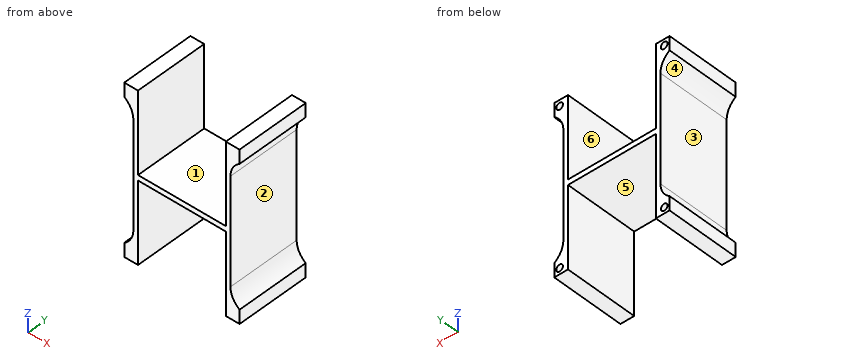
```python
from build123d import *

# Parameters (mm, degrees)
ESQUISSE1_W                  = 43
ESQUISSE1_H                  = 43
BOSS_EXTRU_1_DEPTH           = 40
ESQUISSE2_W                  = 48
ESQUISSE2_H                  = 48
BOSS_EXTRU_2_DEPTH           = 1.5
ENL_V_MAT_EXTRU_3_REACH      = 79.293
ESQUISSE5_W                  = 8
ESQUISSE5_H                  = 5
ENL_V_MAT_EXTRU_4_REACH      = 78.569
ESQUISSE6_W                  = 54.781223227
ESQUISSE6_H                  = 3.078773465
ENL_V_MAT_EXTRU_5_DEPTH      = 9.5
ENL_V_MAT_EXTRU_6_DEPTH      = 73.216687822
ENL_V_MAT_EXTRU_6_DEPTH_BACK = 73.216687822
ESQUISSE9_W                  = 82.255914314
ESQUISSE9_H                  = 90.950558943
ENL_V_MAT_EXTRU_7_DEPTH      = 9.5
ESQUISSE10_W                 = 6
ESQUISSE10_H                 = 36
BOSS_EXTRU_3_DEPTH           = 6
CONG_1_R                     = 10
ESQUISSE11_W                 = 6
ESQUISSE11_H                 = 36
BOSS_EXTRU_4_DEPTH           = 6
CONG_2_R                     = 10
ESQUISSE12_R                 = 1.66
ENL_V_MAT_EXTRU_8_DEPTH      = 10
ESQUISSE13_W                 = 5.657897309
ESQUISSE13_H                 = 15.126215254
ENL_V_MAT_EXTRU_9_DEPTH      = 77.139674284


with BuildPart() as part:
    # Esquisse1 → Boss.-Extru.1 (new body)
    with BuildSketch(Plane.XY):
        Polygon((-2.5, 43), (-2.5, -2.5), (0, -2.5), (45.5, -2.5), (45.5, 43), (45.5, 45.5), (-2.5, 45.5), align=None)
        with Locations((21.5, 21.5)):
            Rectangle(ESQUISSE1_W, ESQUISSE1_H, mode=Mode.SUBTRACT)
    extrude(amount=BOSS_EXTRU_1_DEPTH)

    # Esquisse2 → Boss.-Extru.2 (add)
    with BuildSketch(Plane.XY):
        with Locations((21.5, 21.5)):
            Rectangle(ESQUISSE2_W, ESQUISSE2_H)
    extrude(amount=-BOSS_EXTRU_2_DEPTH)

    # Esquisse5 → Enlèv. mat.-Extru.3 (cut, up to next)
    with BuildSketch(Plane(origin=(0, 45.5, 0), x_dir=(1, 0, 0), z_dir=(0, 1, 0)), mode=Mode.PRIVATE) as enl_v_mat_extru_3_sk1:
        with Locations((21.5, -6.3)):
            Rectangle(ESQUISSE5_W, ESQUISSE5_H)
    enl_v_mat_extru_3_tool1 = extrude(enl_v_mat_extru_3_sk1.sketch, amount=-ENL_V_MAT_EXTRU_3_REACH, mode=Mode.PRIVATE) & part.part
    add(enl_v_mat_extru_3_tool1.solids().sort_by_distance((21.5, 45.5, 6.3))[0], mode=Mode.SUBTRACT)

    # Esquisse6 → Enlèv. mat.-Extru.4 (cut, up to next)
    with BuildSketch(Plane.XY.offset(40), mode=Mode.PRIVATE) as enl_v_mat_extru_4_sk1:
        with Locations((23.162986277, -1.539386733)):
            Rectangle(ESQUISSE6_W, ESQUISSE6_H)
    enl_v_mat_extru_4_tool1 = extrude(enl_v_mat_extru_4_sk1.sketch, amount=-ENL_V_MAT_EXTRU_4_REACH, mode=Mode.PRIVATE) & part.part
    add(enl_v_mat_extru_4_tool1.solids().sort_by_distance((23.162986, -1.539387, 40))[0], mode=Mode.SUBTRACT)

    # Symétrie1: part across plane


with BuildPart() as part_1:
    add(part.part)
    add(part.part.mirror(Plane.XY.offset(-1.5)))

    # Esquisse7 → Enlèv. mat.-Extru.5 (cut)
    with BuildSketch(Plane(origin=(0, 45.5, 0), x_dir=(1, 0, 0), z_dir=(0, 1, 0))):
        Polygon((-2.5, 7.8), (0, 7.8), (0, 12.8), (-2.5, 12.8), (-2.5, 25.4), (0, 25.4), (0, 30.4), (-2.5, 30.4), (-2.5, 43), (45.5, 43), (45.5, 30.4), (43, 30.4), (43, 25.4), (45.5, 25.4), (45.5, 12.8), (43, 12.8), (43, 7.8), (45.5, 7.8), (45.5, -4.8), (43, -4.8), (43, -9.8), (45.5, -9.8), (45.5, -22.4), (43, -22.4), (43, -27.4), (45.5, -27.4), (45.5, -40), (-2.5, -40), (-2.5, -27.4), (0, -27.4), (0, -22.4), (-2.5, -22.4), (-2.5, -9.8), (0, -9.8), (0, -4.8), (-2.5, -4.8), align=None)
    extrude(amount=-ENL_V_MAT_EXTRU_5_DEPTH, mode=Mode.SUBTRACT)

    # Esquisse8 → Enlèv. mat.-Extru.6 (cut, two sides: drawn at the far end of the back side and taken through both)
    with BuildSketch(Plane(origin=(0, 36, 0), x_dir=(1, 0, 0), z_dir=(0, 1, 0)).offset(-ENL_V_MAT_EXTRU_6_DEPTH_BACK)):
        Polygon((-0.2, 43), (-0.2, 2.8), (43.2, 2.8), (43.2, 43), (43, 43), (43, 3), (0, 3), (0, 43), align=None)
        Polygon((0, 0), (0, -40), (-0.2, -40), (-0.2, 0.2), (43.2, 0.2), (43.2, -40), (43, -40), (43, 0), align=None)
    extrude(amount=ENL_V_MAT_EXTRU_6_DEPTH + ENL_V_MAT_EXTRU_6_DEPTH_BACK, mode=Mode.SUBTRACT)

    # Esquisse9 → Enlèv. mat.-Extru.7 (cut)
    with BuildSketch(Plane(origin=(0, 45.5, 0), x_dir=(1, 0, 0), z_dir=(0, 1, 0))):
        with Locations((21.348833146, 1.614403219)):
            Rectangle(ESQUISSE9_W, ESQUISSE9_H)
    extrude(amount=-ENL_V_MAT_EXTRU_7_DEPTH, mode=Mode.SUBTRACT)

    # Esquisse10 → Boss.-Extru.3 (add)
    with BuildSketch(Plane(origin=(45.5, 0, 0), x_dir=(0, 0, -1), z_dir=(1, 0, 0))):
        with Locations((-37, 18)):
            Rectangle(ESQUISSE10_W, ESQUISSE10_H)
        with Locations((40, 18)):
            Rectangle(ESQUISSE10_W, ESQUISSE10_H)
    extrude(amount=BOSS_EXTRU_3_DEPTH)

    # Congé1
    # the kernel refuses this fillet: 10 mm, written as the material it adds along each edge
    with BuildSketch(Plane(origin=(45.5, 36, 34), x_dir=(1, 0, 0), z_dir=(0, -1, 0))) as cong_1_piece_1:
        with BuildLine():
            CenterArc((10, -9.16515139), CONG_1_R, 113.578178478, 66.421821522)
            Line((0, -9.16515139), (-0.2, -9.16515139))
            Line((-0.2, -9.16515139), (-0.2, 0))
            Line((-0.2, 0), (0, 0.2))
            ThreePointArc((0, 0.2), (3, 0.2), (5.92, 0.183303028))
            Line((5.92, 0.183303028), (6, 0))
        make_face()
    extrude(amount=36)
    with BuildSketch(Plane(origin=(45.5, 36, -37), x_dir=(0, 0, 1), z_dir=(0, -1, 0))) as cong_1_piece_2:
        with BuildLine():
            CenterArc((9.16515139, -10), CONG_1_R, 90, 66.421821522)
            Line((0, -6), (-0.183303028, -5.92))
            ThreePointArc((-0.183303028, -5.92), (-0.2, -3), (-0.2, 0))
            Line((-0.2, 0), (0, 0.2))
            Line((0, 0.2), (9.16515139, 0.2))
            Line((9.16515139, 0.2), (9.16515139, 0))
        make_face()
    extrude(amount=36)

    # Esquisse11 → Boss.-Extru.4 (add)
    with BuildSketch(Plane.ZY.offset(2.5)):
        with Locations((-40, 18)):
            Rectangle(ESQUISSE11_W, ESQUISSE11_H)
        with Locations((37, 18)):
            Rectangle(ESQUISSE11_W, ESQUISSE11_H)
    extrude(amount=BOSS_EXTRU_4_DEPTH)

    # Congé2
    # the kernel refuses this fillet: 10 mm, written as the material it adds along each edge
    with BuildSketch(Plane(origin=(-2.5, 0, 34), x_dir=(-1, 0, 0), z_dir=(0, 1, 0))) as cong_2_piece_1:
        with BuildLine():
            CenterArc((10, -9.16515139), CONG_2_R, 113.578178478, 66.421821522)
            Line((0, -9.16515139), (-0.2, -9.16515139))
            Line((-0.2, -9.16515139), (-0.2, 0))
            Line((-0.2, 0), (0, 0.2))
            ThreePointArc((0, 0.2), (3, 0.2), (5.92, 0.183303028))
            Line((5.92, 0.183303028), (6, 0))
        make_face()
    extrude(amount=36)
    with BuildSketch(Plane(origin=(-2.5, 36, -37), x_dir=(0, 0, 1), z_dir=(0, -1, 0))) as cong_2_piece_2:
        with BuildLine():
            CenterArc((9.16515139, 10), CONG_2_R, 203.578178478, 66.421821522)
            Line((0, 6), (-0.183303028, 5.92))
            ThreePointArc((-0.183303028, 5.92), (-0.2, 3), (-0.2, 0))
            Line((-0.2, 0), (0, -0.2))
            Line((0, -0.2), (9.16515139, -0.2))
            Line((9.16515139, -0.2), (9.16515139, 0))
        make_face()
    extrude(amount=36)

    # Esquisse12 → Enlèv. mat.-Extru.8 (cut)
    with BuildSketch(Plane(origin=(0, 36, 0), x_dir=(1, 0, 0), z_dir=(0, 1, 0))):
        with Locations(Location((-4.35, 40, 0), (0, 0, 180))):
            Circle(ESQUISSE12_R)
        with Locations((47.35, 40)):
            Circle(ESQUISSE12_R)
        with Locations(Location((47.35, -37, 0), (0, 0, 180))):
            Circle(ESQUISSE12_R)
        with Locations((-4.35, -37)):
            Circle(ESQUISSE12_R)
    extrude(amount=-ENL_V_MAT_EXTRU_8_DEPTH, mode=Mode.SUBTRACT)

    # Esquisse13 → Enlèv. mat.-Extru.9 (cut, through all)
    with BuildSketch(Plane(origin=(0, 36, 0), x_dir=(1, 0, 0), z_dir=(0, 1, 0))):
        with Locations((52.828948655, 38.373658998)):
            Rectangle(ESQUISSE13_W, ESQUISSE13_H)
        with Locations((52.828948655, -35.373658998)):
            Rectangle(ESQUISSE13_W, ESQUISSE13_H)
        with Locations((-9.828948654, 38.373658998)):
            Rectangle(ESQUISSE13_W, ESQUISSE13_H)
        with Locations((-9.828948654, -35.373658998)):
            Rectangle(ESQUISSE13_W, ESQUISSE13_H)
    extrude(amount=-ENL_V_MAT_EXTRU_9_DEPTH, mode=Mode.SUBTRACT)


solid = part_1.part
```
Can you work these out from the model? Positions are in its coordinate system, mm. Face numbers are marked on the shaded views. A direction names the side the tool comes from. Give positions to 0.01 mm unless a question says otherwise; leave off trailing zeros. Loops run counter-clockwise (first coordinate to the right, second up) from the corner with the lowest first, then second, coordinate; pieces in that order, holes last. Notation, with made-up numbers: M 27.5,78.25 L 57.5,78.25 A15 cw 57.5,89.25 Z; hole C 89,18.25 d4. An arc over 180 degrees is marked long. Use one line per item in the form item = value. Start each with the question number.
(1) I want a section at D-D, the plane z = -16. Write out the boundary of the cut face in (x, y), and give its area (3 significant figures).
(2) I want a section at B-B, the plane x = -4.35. Write out the boundary of the cut face in (y, z).
(3) I want a section at A-A, the plane z = 37. Write out the boundary of the cut face in (x, y).
(4) Thinking about a two-plate mould opening in X: for the marked faces 1, 2 and 3, which applies, released by +X, released by -X, zero draft, split by the parting line, or undercut?
(5) On a 3-axis mill with a long thin cutter (end or side, diameter ignored), from which of +Z, -Z, +X, -X, +Y, -Y can I reach the whole of each face in a straight line? I mean the marked faces 4, 5 and 6. Say none if no direction works.
(6) I want a section at C-C, the plane y = 10.5. Write out the boundary of the cut face in (x, z).
(7) Please list where these lines run through material, in increasing order: line 1 (X direction, y = 10.5, z = 11.5); line 2 (Z direction, x = 47, y = 31); line 3 (Z direction, x = -4.35, y = 28).
(8) I'm going to push flat-ended pins straight in: P1, Ø4, axis at x = 34.5, y = 11.5, coming from the -Z side; P2, Ø2.5, axis at x = -4.35, z = 37, coming from the +Y side; P3, Ø18, axis at y = 12.5, z = -15.5, coming from the -X side. Where does each tip first touch, or does it pass through?
Worked out:
q1.outline = M -2.5,0 L -0.2,0 L -0.2,36 L -2.5,36 Z; M 43.2,0 L 45.5,0 L 45.5,36 L 43.2,36 Z
q1.area = 166 mm²
q2.outline = M 0,-43 L 36,-43 L 36,-41.66 L 26,-41.66 L 26,-38.34 L 36,-38.34 L 36,-33.63 L 0,-33.63 Z; M 0,30.63 L 36,30.63 L 36,35.34 L 26,35.34 L 26,38.66 L 36,38.66 L 36,40 L 0,40 Z
q3.outline = M -7,0 L -0.2,0 L -0.2,36 L -2.69,36 L -2.69,26 L -6.01,26 L -6.01,36 L -7,36 Z; M 43.2,0 L 50,0 L 50,36 L 49.01,36 L 49.01,26 L 45.69,26 L 45.69,36 L 43.2,36 Z
q4.face_1 = undercut
q4.face_2 = released by +X
q4.face_3 = released by -X
q5.face_4 = -X, +Y, -Y
q5.face_5 = -Z, +Y, -Y
q5.face_6 = +Z, +Y, -Y
q6.outline = M -7,-43 L -0.2,-43 L -0.2,-2.8 L 43.2,-2.8 L 43.2,-43 L 50,-43 L 50,-36.19 A10 cw 45.5,-27.83 L 45.5,24.83 A10 cw 50,33.19 L 50,40 L 43.2,40 L 43.2,-0.2 L -0.2,-0.2 L -0.2,40 L -7,40 L -7,33.19 A10 cw -2.5,24.83 L -2.5,-27.83 A10 cw -7,-36.19 Z
q7.line_1 = -2.5 to -0.2, 43.2 to 45.5
q7.line_2 = -43 to -41.62, -38.38 to -33.1, 30.1 to 35.38, 38.62 to 40
q7.line_3 = -43 to -41.66, -38.34 to -33.63, 30.63 to 35.34, 38.66 to 40
q8.P1 = -2.8
q8.P2 = 26
q8.P3 = -2.5
